For this review, take the finished solid that the model builds, in its own axes (mm). Face numbers are marked on the shaded views. A direction names the side the tool comes from. Round coordinates to 2 decimals unless told otherwise and drop trailing zeros. Order: outer loops, then holes, each group sorted by start corner. A loop starts at its lowest first (then second) coordinate and runs counter-clockwise, first axis right, second up. Notation, with made-up numbers: M 50.5,56 L 73.5,56 A19 ccw 73.5,75 Z; hole C 21.5,69 d6. An arc over 180 degrees is marked long. Answer in a Markdown table with one row per item. Add a question column.
```python
from build123d import *

# Parameters (mm, degrees)
SKETCH_3_W          = 19.1
SKETCH_3_H          = 7.03
EXTRUDE_2_DEPTH     = 9.6
SKETCH_7_W          = 19.1
SKETCH_7_H          = 5.03
CUT_EXTRUDE_2_DEPTH = 6.5
SKETCH_8_R          = 0.3
EXTRUDE_4_DEPTH     = 19.1
SKETCH_11_W         = 0.8
SKETCH_11_H         = 3.43
CUT_EXTRUDE_4_DEPTH = 0.8
CUT_EXTRUDE_4_DRAFT = -20
SKETCH_12_W         = 0.8
SKETCH_12_H         = 3.43
CUT_EXTRUDE_5_DEPTH = 0.8
CUT_EXTRUDE_5_DRAFT = -20


with BuildPart() as part:
    # Эскиз3 → Бобышка-Вытянуть2 (new body)
    with BuildSketch(Plane.XY):
        Rectangle(SKETCH_3_W, SKETCH_3_H)
    extrude(amount=EXTRUDE_2_DEPTH)

    # Эскиз7 → Вырез-Вытянуть2 (cut)
    with BuildSketch(Plane(origin=(0, 0, 0), x_dir=(-1, 0, 0), z_dir=(0, 0, -1))):
        Rectangle(SKETCH_7_W, SKETCH_7_H)
    extrude(amount=-CUT_EXTRUDE_2_DEPTH, mode=Mode.SUBTRACT)

    # Эскиз8 → Бобышка-Вытянуть4 (add)
    with BuildSketch(Plane(origin=(9.55, 0, 0), x_dir=(0, 0, -1), z_dir=(1, 0, 0))):
        with Locations((-1, -3.515)):
            Circle(SKETCH_8_R)
        with Locations((-1, 3.515)):
            Circle(SKETCH_8_R)
    extrude(amount=-EXTRUDE_4_DEPTH)


with BuildPart() as cut_extrude_4_tool:
    # Эскиз11 → Вырез-Вытянуть4 (with draft: the straight prism first)
    with BuildSketch(Plane(origin=(9.55, 0, 0), x_dir=(0, 0, -1), z_dir=(1, 0, 0))):
        with Locations((-8.4, 0)):
            Rectangle(SKETCH_11_W, SKETCH_11_H)
    extrude(amount=-CUT_EXTRUDE_4_DEPTH)
    # Вырез-Вытянуть4: the draft: its side faces are tilted about the plane it starts from
    cut_extrude_4_sides = [cut_extrude_4_tool.faces().sort_by_distance(p)[0] for p in [
        (9.15, 0, 8.8),
        (9.15, -1.715, 8.4),
        (9.15, 0, 8),
        (9.15, 1.715, 8.4),
    ]]
    draft(cut_extrude_4_sides, Plane(origin=(9.55, 0, 0), x_dir=(0, 0, -1), z_dir=(1, 0, 0)), CUT_EXTRUDE_4_DRAFT)


with BuildPart() as part_1:
    add(part.part)

    # Вырез-Вытянуть4: cut by cut_extrude_4_tool
    add(cut_extrude_4_tool.part, mode=Mode.SUBTRACT)


with BuildPart() as cut_extrude_5_tool:
    # Эскиз12 → Вырез-Вытянуть5 (with draft: the straight prism first)
    with BuildSketch(Plane.ZY.offset(9.55)):
        with Locations((8.4, 0)):
            Rectangle(SKETCH_12_W, SKETCH_12_H)
    extrude(amount=-CUT_EXTRUDE_5_DEPTH)
    # Вырез-Вытянуть5: the draft: its side faces are tilted about the plane it starts from
    cut_extrude_5_sides = [cut_extrude_5_tool.faces().sort_by_distance(p)[0] for p in [
        (-9.15, 0, 8),
        (-9.15, -1.715, 8.4),
        (-9.15, 0, 8.8),
        (-9.15, 1.715, 8.4),
    ]]
    draft(cut_extrude_5_sides, Plane.ZY.offset(9.55), CUT_EXTRUDE_5_DRAFT)


with BuildPart() as part_2:
    add(part_1.part)

    # Вырез-Вытянуть5: cut by cut_extrude_5_tool
    add(cut_extrude_5_tool.part, mode=Mode.SUBTRACT)


solid = part_2.part
```
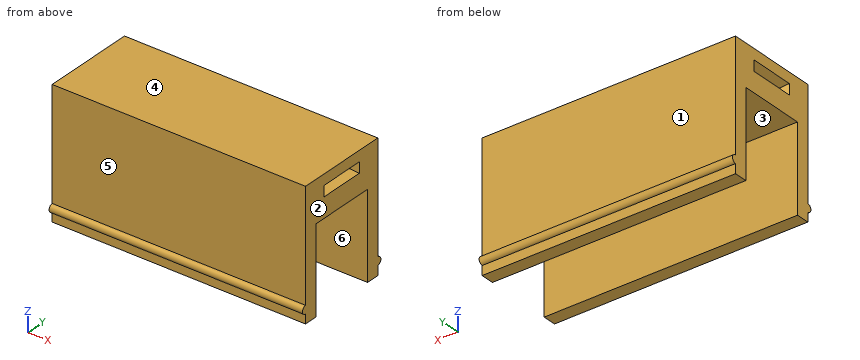
1. Clearance check with flat-ended pins moving along their axes: pin 1 Ø2.5 at (x, z) = (-1.5, 7) entering from +Y (3 decimals); pin 2 Ø5 at (x, z) = (1.5, 4.5) entering from -Y (3 decimals). State where each tip first meets the part, or that it passes through.
2. The part is to be moulded in two halves that separate along Y. For the marked faces 1, 2 and 3, say which applies: pulls with the +Y half, pulls with the -Y half, needs draft (parallel to the pull), parting line crosses it, or undercut.
3. To check wall thickness, follow probe 1 along Y at (x, z) = (0, 3.5) (3 decimals); probe 2 along Y at (x, z) = (-4.5, 1) (3 decimals); probe 3 along Y at (x, z) = (-0.5, 9) (3 decimals). State the ranges of each line that lie inside material, in increasing order. Write a range as [from, to].
4. Consider section B-B on x = -8. Write out the cut boundary in (y, z) (3 decimals), plus the area to 3 significant figures.
5. Consider section D-D on z = 9.25. Write out the cut boundary in (x, y) (3 decimals).
6. Consider section C-C on z = 1. Write out the cut boundary in (x, y) (3 decimals).
7. For the marked faces 4, 5 and 6, list the 3-axis set-ups (+Z, -Z, +X, -X, +Y, -Y) from which the entire face can be reached by the end or side of a thin tool; tool diameter is ignored.
8. Consider section A-A on z = 4.5. Write out the cut boundary in (x, y) (3 decimals), plus the area to 3 significant figures.
Solved:
| question | item | result |
|---|---|---|
| 1 | pin 1 | stops at y = 3.515 |
| 1 | pin 2 | stops at y = -3.515 |
| 2 | face 1 | pulls with the +Y half |
| 2 | face 2 | needs draft |
| 2 | face 3 | undercut |
| 3 | probe 1 | y = [-3.515, -2.515], [2.515, 3.515] |
| 3 | probe 2 | y = [-3.815, -2.515], [2.515, 3.815] |
| 3 | probe 3 | y = [-3.515, 3.515] |
| 4 | outline | M -3.515,0 L -2.515,0 L -2.515,6.5 L 2.515,6.5 L 2.515,0 L 3.515,0 L 3.515,0.7 A0.3 ccw 3.515,1.3 L 3.515,9.6 L -3.515,9.6 L -3.515,1.3 A0.3 ccw -3.515,0.7 Z |
| 4 | area | 35.1 mm^2 |
| 5 | outline | M -9.55,-3.515 L 9.55,-3.515 L 9.55,3.515 L -9.55,3.515 Z |
| 6 | outline | M -9.55,-3.815 L 9.55,-3.815 L 9.55,-2.515 L -9.55,-2.515 Z; M -9.55,2.515 L 9.55,2.515 L 9.55,3.815 L -9.55,3.815 Z |
| 7 | face 4 | +Z, +X, -X, +Y, -Y |
| 7 | face 5 | +Z, +X, -X, -Y |
| 7 | face 6 | -Z, +X, -X |
| 8 | outline | M -9.55,-3.515 L 9.55,-3.515 L 9.55,-2.515 L -9.55,-2.515 Z; M -9.55,2.515 L 9.55,2.515 L 9.55,3.515 L -9.55,3.515 Z |
| 8 | area | 38.2 mm^2 |
